Geometry check sheet. Reference: the model listing, model coordinates, mm. Round coordinates to 2 decimals unless told otherwise and drop trailing zeros. Order: outer loops, then holes, each group sorted by start corner. A loop starts at its lowest first (then second) coordinate and runs counter-clockwise, first axis right, second up.
(1) Go/stop test with flat-tipped pins: pin 1 (4 mm diameter, centred on y = 5, z = -2.5, fed in from +X); pin 2 (0.8 mm diameter, centred on x = 19.5, z = -0.5, fed in from +Y); pin 3 (0.8 mm diameter, centred on x = 44.5, y = -38.5, fed in from -Z). Record where each tip stops, or that it passes through.
(2) Sectioned sample at B-B (x = 36). Record the boundary of the cut face in (y, z), plus the area to 3 significant figures.
(3) Sectioned sample at C-C (y = 2). Record the boundary of the cut face in (x, z), plus the area to 3 significant figures.
(4) Sectioned sample at A-A (y = -26). Record the boundary of the cut face in (x, z).
(5) Material ranges on line 1 along X through (y, z) = (41.5, 2.5); line 2 along Y through (x, z) = (58.6, 2.85); line 3 along Z through (x, y) = (70.5, 41), recorded low to high.
(6) Sectioned sample at D-D (x = -4.4). Record the boundary of the cut face in (y, z).
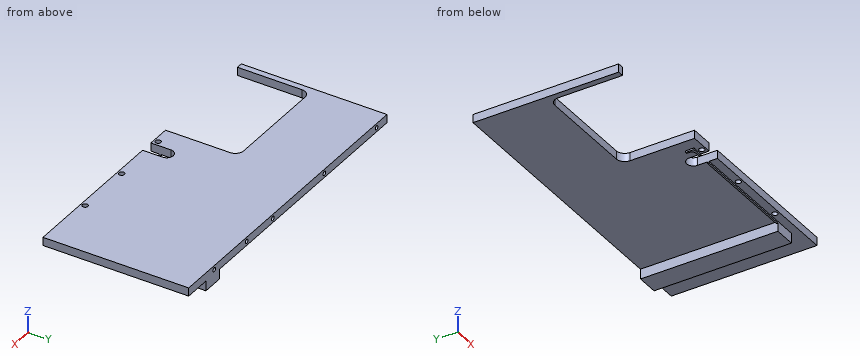
from build123d import *

# Parameters (mm, degrees)
SKETCH1_W              = 190
SKETCH1_H              = 88
BOSS_EXTRUDE1_DEPTH    = 5
SKETCH2_W              = 13
SKETCH2_H              = 83
BOSS_EXTRUDE2_DEPTH    = 6
BOSS_EXTRUDE3_DEPTH    = 1
SKETCH7_R              = 1.65
CUT_EXTRUDE3_DEPTH     = 6
FILLET3_R              = 2
HOLE_WIZARD_M3_1_D     = 2.5
HOLE_WIZARD_M3_1_DEPTH = 8.5
HOLE_WIZARD_M3_1_TIP   = 0.751075774
CUT_EXTRUDE_START      = -5
CUT_EXTRUDE_1_DEPTH    = 12
SKETCH_4_W             = 68.9
SKETCH_4_H             = 44
CUT_EXTRUDE_2_DEPTH    = 12
FILLET_1_R             = 5


with BuildPart() as part:
    # Sketch1 → Boss-Extrude1 (new body)
    with BuildSketch(Plane.XY):
        Rectangle(SKETCH1_W, SKETCH1_H)
    extrude(amount=BOSS_EXTRUDE1_DEPTH)

    # Sketch2 → Boss-Extrude2 (add)
    with BuildSketch(Plane(origin=(0, 0, 0), x_dir=(-1, 0, 0), z_dir=(0, 0, -1))):
        with Locations((-72, 2.5)):
            Rectangle(SKETCH2_W, SKETCH2_H)
    extrude(amount=BOSS_EXTRUDE2_DEPTH)

    # Sketch4 → Boss-Extrude3 (add)
    with BuildSketch(Plane(origin=(0, 0, 0), x_dir=(-1, 0, 0), z_dir=(0, 0, -1))):
        Polygon((-65.5, -38), (14, -38), (14, -34), (15, -34), (15, -39), (-65.5, -39), align=None)
    extrude(amount=BOSS_EXTRUDE3_DEPTH)

    # Sketch7 → Cut-Extrude3 (cut, through all)
    with BuildSketch(Plane(origin=(0, 0, 0), x_dir=(-1, 0, 0), z_dir=(0, 0, -1))):
        with Locations((-58.6, -41.5)):
            Circle(SKETCH7_R)
        with Locations((-23.6, -41.5)):
            Circle(SKETCH7_R)
        with Locations((11.4, -41.5)):
            Circle(SKETCH7_R)
    extrude(amount=-CUT_EXTRUDE3_DEPTH, mode=Mode.SUBTRACT)

    # Fillet3
    fillet3_edges = [part.edges().sort_by_distance(p)[0] for p in [
        (-14, -38, -0.5),
    ]]
    fillet(fillet3_edges, radius=FILLET3_R)

    # M3 螺纹孔1
    with Locations(Plane(origin=(-85, 44, 2.5), x_dir=(0, 0, 1), z_dir=(0, 1, 0))):
        with Locations((0, 0), (0, 50), (0, 99.373308098), (0, 124.5), (0, 155.5)):
            Hole(HOLE_WIZARD_M3_1_D / 2, depth=HOLE_WIZARD_M3_1_DEPTH)
            with Locations((0, 0, -(HOLE_WIZARD_M3_1_DEPTH + HOLE_WIZARD_M3_1_TIP / 2))):  # 118° drill point
                Cone(0, HOLE_WIZARD_M3_1_D / 2, HOLE_WIZARD_M3_1_TIP, mode=Mode.SUBTRACT)

    # 草图3 → 切除-拉伸1 (cut, through all)
    with BuildSketch(Plane(origin=(0, 0, 0), x_dir=(-1, 0, 0), z_dir=(0, 0, -1)).offset(CUT_EXTRUDE_START)):
        with BuildLine():
            Line((0.4, -44), (0.4, -32))
            ThreePointArc((0.4, -32), (4.4, -28), (8.4, -32))
            Line((8.4, -32), (8.4, -44))
            Line((8.4, -44), (0.4, -44))
        make_face()
    extrude(amount=CUT_EXTRUDE_1_DEPTH, mode=Mode.SUBTRACT)

    # 草图4 → 切除-拉伸2 (cut, through all)
    with BuildSketch(Plane.XY.offset(5)):
        with Locations((-56.85, -22)):
            Rectangle(SKETCH_4_W, SKETCH_4_H)
    extrude(amount=-CUT_EXTRUDE_2_DEPTH, mode=Mode.SUBTRACT)

    # 圆角1
    fillet_1_edges = [part.edges().sort_by_distance(p)[0] for p in [
        (-91.3, 0, 2.5),
        (-22.4, 0, 2.5),
    ]]
    fillet(fillet_1_edges, radius=FILLET_1_R)


solid = part.part
Answer below:
1. pin 1: stops at x = 78.5
1. pin 2: stops at y = -38
1. pin 3: stops at z = -1
2. outline: (-44, 0) - (-39, 0) - (-39, -1) - (-38, -1) - (-38, 0) - (44, 0) - (44, 5) - (-44, 5) - close
2. area: 441 mm2
3. outline: (-95, 0) - (65.5, 0) - (65.5, -6) - (78.5, -6) - (78.5, 0) - (95, 0) - (95, 5) - (-95, 5) - close
3. area: 1,030 mm2
4. outline: (-95, 0) - (-91.3, 0) - (-91.3, 5) - (-95, 5) - close; (-22.4, 0) - (65.5, 0) - (65.5, -6) - (78.5, -6) - (78.5, 0) - (95, 0) - (95, 5) - (-22.4, 5) - close
5. line 1: x = -95 to -86.25, -83.75 to -36.25, -33.75 to 13.12, 15.62 to 38.25, 40.75 to 69.25, 71.75 to 95
5. line 2: y = -44 to -43.15, -39.85 to 44
5. line 3: z = -6 to 1.25, 3.75 to 5
6. outline: (-28, 0) - (44, 0) - (44, 5) - (-28, 5) - close
